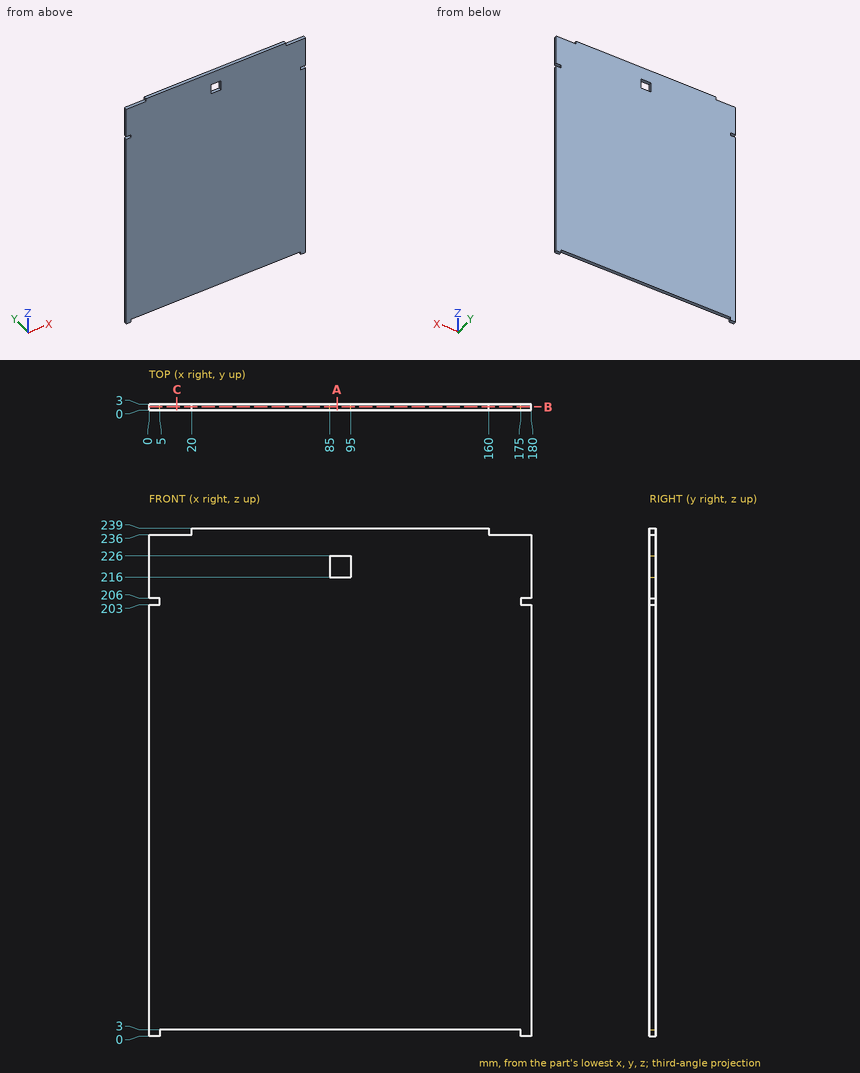
Can you work these out from the drawing? Everything is in mm from the part's minimum corner. Round coordinates to 2 decimals unless told otherwise and drop trailing zeros. Loops run counter-clockwise (first coordinate to the right, second up) from the corner with the lowest first, then second, coordinate; pieces in that order, holes last. Notation, with made-up numbers: (-23.75, 52.25) - (1.25, 52.25) arc R18 ccw to (1.25, 70.25) - close; hole circle Ø2 at (49.25, 11.5). An arc over 180 degrees is marked (long way). Answer in a Markdown table with one row per item. Add a question column.
Q1. I want a section at B-B on y = 1.6. List the corners of the cut face in (x, z) for me, and give its area (3 significant figures).
Q2. For pin 1 Ø0.9 at (x, y) = (89.5, 1.5) entering from -Z; pin 2 Ø12 at (x, z) = (137.5, 126.5) entering from -Y; pin 3 Ø1.5 at (y, z) = (2, 205) entering from +X; pin 4 Ø1.5 at (x, y) = (2, 2) entering from +Z, each with a flat end and sliding along its axis, tell me the tip position at first contact or that it passes through.
Q3. I need wall thicknesses on L1, parallel to Z at x = 170, y = 0.85; L2, parallel to Z at x = 88.5, y = 1.4; L3, parallel to Z at x = 54, y = 0.5. Which ranges of each line are inside material? Lowest first, please.
Q4. I want a section at C-C on x = 13. List the corners of the cut face in (y, z) for me, and give its area (3 significant figures).
Q5. I want a section at A-A on x = 88.5. List the corners of the cut face in (y, z) for me, and give its area (3 significant figures).
A:
| question | item | result |
|---|---|---|
| 1 | outline | (0, 0) - (5, 0) - (5, 3) - (175, 3) - (175, 0) - (180, 0) - (180, 203) - (175, 203) - (175, 206) - (180, 206) - (180, 236) - (160, 236) - (160, 239) - (20, 239) - (20, 236) - (0, 236) - (0, 206) - (5, 206) - (5, 203) - (0, 203) - close; hole (85, 216) - (95, 216) - (95, 226) - (85, 226) - close |
| 1 | area | 42,300 mm^2 |
| 2 | pin 1 | z = 3 |
| 2 | pin 2 | y = 0 |
| 2 | pin 3 | x = 175 |
| 2 | pin 4 | z = 236 |
| 3 | L1 | 3 to 236 |
| 3 | L2 | 3 to 216, 226 to 239 |
| 3 | L3 | 3 to 239 |
| 4 | outline | (0, 3) - (3, 3) - (3, 236) - (0, 236) - close |
| 4 | area | 699 mm^2 |
| 5 | outline | (0, 3) - (3, 3) - (3, 216) - (0, 216) - close; (0, 226) - (3, 226) - (3, 239) - (0, 239) - close |
| 5 | area | 678 mm^2 |
